Autodesk Inventor part; units mm, degrees
ref_plane "YZ Plane" through (0, 0, 0) normal (1, 0, 0) x (0, 1, 0)
ref_plane "XZ Plane" through (0, 0, 0) normal (0, 1, 0) x (-1, 0, 0)
ref_plane "XY Plane" through (0, 0, 0) normal (0, 0, 1) x (1, 0, 0)
sketch "スケッチ1" plane through (0, 0, 0) normal (0, 0, 1) x (1, 0, 0)
  circle A0 centre (0, 0) radius 5
  dimension "d0" = 10
extrude "押し出し1" add sketch "スケッチ1" along normal blind 0.3
sketch "スケッチ2" plane through (0, 0, 0.3) normal (0, 0, 1) x (1, 0, 0)
  circle A0 centre (0, 0) radius 2.5
  dimension "d3" = 5
extrude "押し出し2" add sketch "スケッチ2" along normal blind 1
sketch "スケッチ3" plane through (0, 0, 1.3) normal (0, 0, 1) x (1, 0, 0)
  point P0 (0, 0)
  point P1 (0, 0)
hole "穴1" at (0, 0, 1.3) direction (0, 0, -1) diameter 3 end through all
properties part number "Φ3軸用プッシュナット"
Can you work these out from the model? Positions are in its coordinate system, mm. A direction names the side the tool comes from. Coordinates: 2 decimals unless noted, no trailing zeros. Loops run counter-clockwise (first coordinate to the right, second up) from the corner with the lowest first, then second, coordinate; pieces in that order, holes last. Notation, with made-up numbers: M -5.5,19 L 50.5,19 A20 ccw 50.5,26 Z; hole C 47,43.25 d10. An arc over 180 degrees is marked long. Return JSON: item names as keys, results as strings. Group by question number.
Item 1: If I drill on L1, parallel to Y at x = 0, z = 0.6; L2, parallel to Y at x = 0, z = 0.1; L3, parallel to X at y = -0.75, z = 0.4, over which ranges is the centre line in solid material (lowest first)? Write a range as from..to.
Item 2: Imagine slicing it at A-A (x = 0). Please give me the cut outline in (y, z), and give its area (3 significant figures).
Item 3: Imagine slicing it at C-C (x = -1.75). Please give me the cut outline in (y, z), and give its area (3 significant figures).
Item 4: On a 3-axis mill with a long thin cutter (end or side, diameter ignored), from which of +Z, -Z, +X, -X, +Y, -Y can I reach the whole of each face in a straight line? I mean faces 1 (the flat face through (2, 0, 1.3)), 2 (the cylindrical face through (-0.54, 2.44, 0.79)). Say none if no direction works.
Item 5: Thinking about a two-plate mould opening in Y: for faces 3 (the cylindrical face through (4.77, -1.5, 0.15)), 4 (the flat face through (-1.2, 1.2, 0)), 5 (the cylindrical face through (-0.07, 1.5, 0.64)), which applies, released by +Y, released by -Y, zero draft, split by the parting line, or undercut?
Item 6: I'm going to push flat-ended pins straight in: pin 1 Ø3.5 at (x, y) = (0, 0) entering from +Z; pin 2 Ø1.5 at (x, y) = (2.5, -3.5) entering from +Z. Where does each tip first touch, or does it pass through?
Item 7: Imagine slicing it at D-D (z = 0.45). Please give me the cut outline in (x, y).
Verdict:
{
 "1": {"L1": "y = -2.5..-1.5, 1.5..2.5", "L2": "y = -5..-1.5, 1.5..5", "L3": "x = -2.38..-1.3, 1.3..2.38"},
 "2": {"outline": "M -5,0 L -1.5,0 L -1.5,1.3 L -2.5,1.3 L -2.5,0.3 L -5,0.3 Z; M 1.5,0 L 5,0 L 5,0.3 L 2.5,0.3 L 2.5,1.3 L 1.5,1.3 Z", "area": "4.10 mm^2"},
 "3": {"outline": "M -4.68,0 L 4.68,0 L 4.68,0.3 L 1.79,0.3 L 1.79,1.3 L -1.79,1.3 L -1.79,0.3 L -4.68,0.3 Z", "area": "6.38 mm^2"},
 "4": {"face 1": "+Z, +X, -X, +Y, -Y", "face 2": "+Z"},
 "5": {"face 3": "split by the parting line", "face 4": "zero draft", "face 5": "undercut"},
 "6": {"pin 1": "stops at z = 1.3", "pin 2": "stops at z = 0.3"},
 "7": {"outline": "C 0,0 d5; hole C 0,0 d3"}
}
